Can you work these out from the model? Positions are in its coordinate system, mm. Face numbers are marked on the shaded views. Round coordinates to 2 decimals unless told otherwise and drop trailing zeros. Order: outer loops, then holes, each group sorted by start corner. A loop starts at its lowest first (then second) coordinate and runs counter-clockwise, first axis right, second up. Notation, with made-up numbers: M -37,65 L 6,65 A22 cw 6,90 Z; hole C 83.5,26 d5. An arc over 180 degrees is marked long. Answer as a JSON object with one key per item and string values. Group by question number.
Autodesk Inventor part; units mm, degrees
ref_plane "YZ Plane" through (0, 0, 0) normal (1, 0, 0) x (0, 1, 0)
ref_plane "XZ Plane" through (0, 0, 0) normal (0, 1, 0) x (-1, 0, 0)
ref_plane "XY Plane" through (0, 0, 0) normal (0, 0, 1) x (1, 0, 0)
sketch "Boceto1" plane through (0, 0, 0) normal (0, 1, 0) x (-1, 0, 0)
  line L0 (2.5, -1.4434) -> (0, -2.8868)
  line L1 (0, -2.8868) -> (-2.5, -1.4434)
  line L2 (-2.5, -1.4434) -> (-2.5, 1.4434)
  line L3 (-2.5, 1.4434) -> (0, 2.8868)
  line L4 (0, 2.8868) -> (2.5, 1.4434)
  line L5 (2.5, 1.4434) -> (2.5, -1.4434)
  point P0 (0, 0)
  point P1 (0, 0)
  dimension "d0" = 5
extrude "Extrusión1" add sketch "Boceto1" along normal blind 30
sketch "Boceto2" plane through (0, 0, 0) normal (0, -1, 0) x (1, 0, 0)
  point P0 (0, 0)
  point P1 (0, 0)
hole "Agujero1" at (0, 0, 0) direction (0, 1, 0) diameter 3 depth 8 tip angle 118 countersink diameter 4 countersink angle 90
sketch "Boceto3" plane through (0, 30, 0) normal (0, 1, 0) x (1, 0, 0)
  circle A0 centre (0, 0) radius 1.5
hole "Agujero2" at (0, 30, 0) direction (0, -1, 0) diameter 3 depth 8 tip angle 118 countersink diameter 4 countersink angle 90
properties part number "Separador M3 x 25 mm"
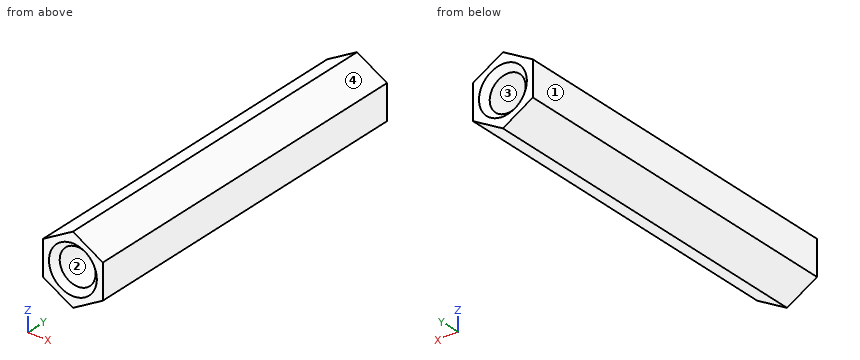
1) If we section it at B-B on y = 15.5: Write out the boundary of the cut face in (x, z).
2) If we section it at A-A on y = 25: Write out the boundary of the cut face in (x, z), plus the area to 3 significant figures.
3) For pin 1 (2.5 mm diameter, centred on x = 0, z = 0, fed in from +Y); pin 2 (1.5 mm diameter, centred on x = 2, y = 23.5, fed in from -Z); pin 3 (2 mm diameter, centred on x = -0.5, y = 6.5, fed in from -Z), each with a flat end and sliding along its axis, tell me the tip position at first contact or that it passes through.
4) We'd pull the mould along Z, two halves only. Please class the marked faces 1, 2, 3 and 4: +Z half, -Z half, draft (parallel to the pull), parting line (faces both ways), or undercut.
5) I need wall thicknesses on line 1 along X through (y, z) = (3.5, 0); line 2 along Z through (x, y) = (0.8, 1.5); line 3 along X through (y, z) = (1.5, 0.8). Which ranges of each line are inside material? Lowest first, please.
Findings:
{
 "1": {"outline": "M -2.5,-1.44 L 0,-2.89 L 2.5,-1.44 L 2.5,1.44 L 0,2.89 L -2.5,1.44 Z"},
 "2": {"outline": "M -2.5,-1.44 L 0,-2.89 L 2.5,-1.44 L 2.5,1.44 L 0,2.89 L -2.5,1.44 Z; hole C 0,0 d3", "area": "14.6 mm^2"},
 "3": {"pin 1": "stops at y = 21.85", "pin 2": "stops at z = -2.17", "pin 3": "stops at z = -2.89"},
 "4": {"face 1": "draft", "face 2": "undercut", "face 3": "undercut", "face 4": "+Z half"},
 "5": {"line 1": "x = -2.5 to -1.5, 1.5 to 2.5", "line 2": "z = -2.42 to -1.27, 1.27 to 2.42", "line 3": "x = -2.5 to -1.27, 1.27 to 2.5"}
}
